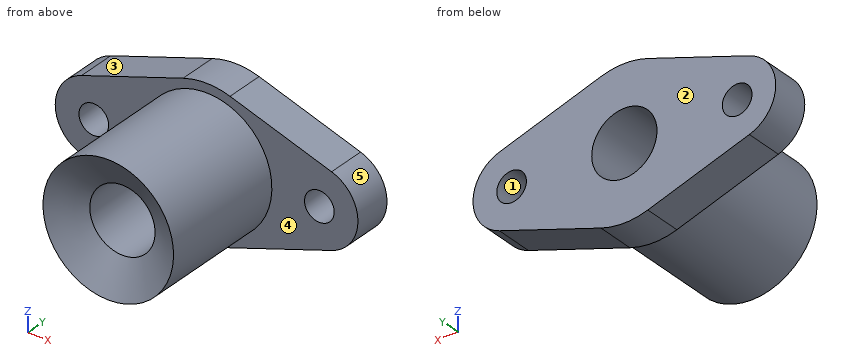
```python
from build123d import *

# Parameters (mm, degrees)
BOSS_EXTRUDE2_START = 13
SKETCH2_R           = 5
SKETCH2_R_2         = 22
SKETCH2_R_3         = 11
BOSS_EXTRUDE2_DEPTH = 13


with BuildPart() as part:
    # Sketch1 → Revolve1 (revolve)
    with BuildSketch(Plane.XY, mode=Mode.PRIVATE) as revolve1_sk:
        Polygon((-22, 0), (-22, 44), (-11, 44), (-11, 6.350852961), align=None)
    revolve(revolve1_sk.sketch.rotate(Axis((0, 0, 0), (0, 1, 0)), 270), axis=Axis((0, 0, 0), (0, 1, 0)))

    # Sketch2 → Boss-Extrude2 (add)
    # profile 1 of 2: a face of its own
    with BuildSketch(Plane(origin=(0, 44, 0), x_dir=(1, 0, 0), z_dir=(0, 1, 0)).offset(BOSS_EXTRUDE2_START)):
        with BuildLine():
            Line((42.109187711, 12.333473815), (7.905910187, 23.729102474))
            ThreePointArc((7.905910187, 23.729102474), (0, 25.01147177), (-7.905910187, 23.729102474))
            Line((-7.905910187, 23.729102474), (-42.109187711, 12.333473815))
            ThreePointArc((-42.109187711, 12.333473815), (-51, 0), (-42.109187711, -12.333473815))
            Line((-42.109187711, -12.333473815), (-7.905910187, -23.729102474))
            ThreePointArc((-7.905910187, -23.729102474), (0, -25.01147177), (7.905910187, -23.729102474))
            Line((7.905910187, -23.729102474), (42.109187711, -12.333473815))
            ThreePointArc((42.109187711, -12.333473815), (51, 0), (42.109187711, 12.333473815))
        make_face()
        with Locations(Location((38, 0, 0), (0, 0, 90))):
            Circle(SKETCH2_R, mode=Mode.SUBTRACT)
        with Locations(Location((-38, 0, 0), (0, 0, 90))):
            Circle(SKETCH2_R, mode=Mode.SUBTRACT)
        with Locations(Location((0, 0, 0), (0, 0, 90))):
            Circle(SKETCH2_R_2, mode=Mode.SUBTRACT)
    # profile 2 of 2: a face of its own
    with BuildSketch(Plane(origin=(0, 44, 0), x_dir=(1, 0, 0), z_dir=(0, 1, 0)).offset(BOSS_EXTRUDE2_START)):
        with Locations(Location((0, 0, 0), (0, 0, 90))):
            Circle(SKETCH2_R_2)
        with Locations(Location((0, 0, 0), (0, 0, 90))):
            Circle(SKETCH2_R_3, mode=Mode.SUBTRACT)
    extrude(amount=-BOSS_EXTRUDE2_DEPTH)


solid = part.part
```
Input: part model. Units: mm. Frame: model coordinates. Face numbers are marked on the shaded views. A direction names the side the tool comes from. Give positions to 0.01 mm unless a question says otherwise; leave off trailing zeros. Write each loop counter-clockwise with the first axis right and the second up, starting at its lowest first coordinate (ties: lowest second). Pieces come first, ordered by that corner, then holes. Notation, with made-up numbers: (61, -26) - (77, -26) arc R18 cw to (77, -20) - close; hole circle Ø10 at (26.25, -11). An arc over 180 degrees is marked (long way). Write item = value, one per line. Start each with the question number.
1. Ray query, L1, parallel to Y at x = -21.5, z = 9; L2, parallel to X at y = 19, z = 0.5; L3, parallel to X at y = 36, z = 8. Return the intervals inside material, ascending.
2. Access query for the marked faces 4 and 5. Directions: +Z, -Z, +X, -X, +Y, -Y. A direction counts if a zero-diameter tool reaches every point of the face in a straight line with its end or side. Return the directions, or none.
3. Section query C-C, the plane y = 21.5. Output: boundary loops of the cut face in (x, z).
4. First-contact query: pin 1 Ø13 at (x, z) = (38, 0) entering from -Y; pin 2 Ø1 at (x, y) = (5, 7.5) entering from -Z; pin 3 Ø10 at (x, y) = (-4.5, 39.5) entering from -Z. Flat tips, straight axial feed; report the tip coordinate or a pass-through.
5. Section query B-B, the plane z = 0. Output: boundary loops of the cut face in (x, y), then the cut area to 3 significant figures.
6. Section query A-A, the plane x = 0. Output: boundary loops of the cut face in (y, z).
7. Mould query, pull axis Z, two halves, no side actions, for the marked faces 1, 2 and 3. Classes: released by +Z, released by -Z, zero draft, split by the parting line, or undercut.
8. Section query D-D, the plane x = -38. Output: boundary loops of the cut face in (y, z).
Check sheet entries:
q1.L1 = 44 to 57
q1.L2 = -21.99 to -10.99, 10.99 to 21.99
q1.L3 = -20.49 to -7.55, 7.55 to 20.49
q2.face_4 = -Y
q2.face_5 = +X, +Y, -Y
q3.outline = circle Ø44 at (0, 0); hole circle Ø22 at (0, 0)
q4.pin_1 = 44
q4.pin_2 = -21.53
q4.pin_3 = -24.9
q5.outline = (-51, 44) - (-43, 44) - (-43, 57) - (-51, 57) - close; (-33, 44) - (-22, 44) - (-22, 0) - (-11, 6.35) - (-11, 57) - (-33, 57) - close; (11, 6.35) - (22, 0) - (22, 44) - (33, 44) - (33, 57) - (11, 57) - close; (43, 44) - (51, 44) - (51, 57) - (43, 57) - close
q5.area = 1,680 mm2
q6.outline = (0, -22) - (44, -22) - (44, -25.01) - (57, -25.01) - (57, -11) - (6.35, -11) - close; (0, 22) - (6.35, 11) - (57, 11) - (57, 25.01) - (44, 25.01) - (44, 22) - close
q7.face_1 = undercut
q7.face_2 = zero draft
q7.face_3 = released by +Z
q8.outline = (44, -13.7) - (57, -13.7) - (57, -5) - (44, -5) - close; (44, 5) - (57, 5) - (57, 13.7) - (44, 13.7) - close
